```python
from build123d import *

# Parameters (mm, degrees)
ESBO_O1_W                            = 100
ESBO_O1_H                            = 40
RESSALTO_EXTRUS_O1_DEPTH             = 10
RESSALTO_EXTRUS_O2_DEPTH             = 10
ESBO_O3_W                            = 39.962527671
ESBO_O3_H                            = 3
CORTE_EXTRUS_O1_DEPTH                = 121.933866224
FILETE1_R                            = 8
FURO_DE_DI_METRO_7_0_7_1_D           = 7
FURO_DE_DI_METRO_7_0_7_1_CSINK_D     = 7.05
FURO_DE_DI_METRO_7_0_7_1_CSINK_ANGLE = 90
FURO_DE_DI_METRO_7_0_7_3_D           = 7
FURO_DE_DI_METRO_7_0_7_3_CSINK_D     = 7.05
FURO_DE_DI_METRO_7_0_7_3_CSINK_ANGLE = 90
FILETE3_R                            = 3


with BuildPart() as part:
    # Esboço1 → Ressalto-extrusão1 (new body)
    with BuildSketch(Plane(origin=(0, 0, 0), x_dir=(1, 0, 0), z_dir=(0, 1, 0))):
        with Locations((50, 20)):
            Rectangle(ESBO_O1_W, ESBO_O1_H)
    extrude(amount=RESSALTO_EXTRUS_O1_DEPTH)

    # Esboço2 → Ressalto-extrusão2 (add)
    with BuildSketch(Plane.XY):
        with BuildLine():
            Line((30, 0), (30, 35))
            ThreePointArc((30, 35), (50, 55), (70, 35))
            Line((70, 35), (70, 0))
            Line((70, 0), (30, 0))
        make_face()
    extrude(amount=-RESSALTO_EXTRUS_O2_DEPTH)

    # Esboço3 → Corte-extrusão1 (cut, through all)
    with BuildSketch(Plane.XY):
        with Locations((50.018736164, 1.5)):
            Rectangle(ESBO_O3_W, ESBO_O3_H)
    extrude(amount=-CORTE_EXTRUS_O1_DEPTH, mode=Mode.SUBTRACT)

    # Filete1
    # the kernel refuses this fillet: 8 mm, written as the material it adds along each edge
    with BuildSketch(Plane(origin=(70, 3, 0), x_dir=(-1, 0, 0), z_dir=(0, 0, -1))) as filete1_piece_1:
        with BuildLine():
            CenterArc((6.244997998, -8), FILETE1_R, 90, 51.317812547)
            Line((0, -3), (0, 0))
            Line((0, 0), (6.244997998, 0))
        make_face()
    extrude(amount=40)
    with BuildSketch(Plane(origin=(30.037472329, 3, 0), x_dir=(0, -1, 0), z_dir=(0, 0, -1))) as filete1_piece_2:
        with BuildLine():
            CenterArc((8, -6.244997998), FILETE1_R, 128.682187453, 51.317812547)
            Line((0, -6.244997998), (0, 0))
            Line((0, 0), (3, 0))
        make_face()
    extrude(amount=40)
    # the kernel refuses this fillet: 8 mm, written as the material it takes off along each edge
    with BuildSketch(Plane(origin=(100, -20, 0), x_dir=(-1, 0, 0), z_dir=(0, 1, 0)), Plane(origin=(100, -20, -40), x_dir=(0, 0, 1), z_dir=(0, 1, 0))) as filete1_2_piece_1:
        with BuildLine():
            CenterArc((FILETE1_R, -FILETE1_R), FILETE1_R, 90, 90)
            Line((0, -FILETE1_R), (0, 0))
            Line((0, 0), (FILETE1_R, 0))
        make_face()
    extrude(amount=50, mode=Mode.SUBTRACT)
    with BuildSketch(Plane(origin=(0, -20, -40), x_dir=(0, 0, 1), z_dir=(0, 1, 0)), Plane(origin=(0, -20, 0), x_dir=(1, 0, 0), z_dir=(0, 1, 0))) as filete1_2_piece_2:
        with BuildLine():
            CenterArc((FILETE1_R, FILETE1_R), FILETE1_R, 180, 90)
            Line((0, FILETE1_R), (0, 0))
            Line((0, 0), (FILETE1_R, 0))
        make_face()
    extrude(amount=50, mode=Mode.SUBTRACT)

    # Furo de diâmetro Ø7.0 (7)1 (through all)
    with Locations(Plane(origin=(0, 10, 0), x_dir=(1, 0, 0), z_dir=(0, 1, 0))):
        with Locations((8, 32)):
            CounterSinkHole(FURO_DE_DI_METRO_7_0_7_1_D / 2, FURO_DE_DI_METRO_7_0_7_1_CSINK_D / 2, counter_sink_angle=FURO_DE_DI_METRO_7_0_7_1_CSINK_ANGLE)

    # Furo de diâmetro Ø7.0 (7)3 (through all)
    with Locations(Plane(origin=(0, 10, 0), x_dir=(1, 0, 0), z_dir=(0, 1, 0))):
        with Locations((92, 32)):
            CounterSinkHole(FURO_DE_DI_METRO_7_0_7_3_D / 2, FURO_DE_DI_METRO_7_0_7_3_CSINK_D / 2, counter_sink_angle=FURO_DE_DI_METRO_7_0_7_3_CSINK_ANGLE)

    # Esboço16 → Rebaixo para parafuso de cabeça sextavada de M81 (revolve, cut)
    with BuildSketch(Plane(origin=(50, 35, 0), x_dir=(0, -1, 0), z_dir=(1, 0, 0))):
        Polygon((0, 0), (0, 40), (4.5, 40), (4.5, 5.68), (9.005, 5.68), (9.005, 0.025), (9.03, 0), align=None)
    revolve(axis=Axis((50, 35, 6.35), (0, 0, -1)), mode=Mode.SUBTRACT)

    # Filete3
    filete3_edges = [part.edges().sort_by_distance(p)[0] for p in [
        (81, 10, 0),
        (30, 22.5, -10),
        (70, 22.5, -10),
        (30, 22.5, 0),
        (70, 22.5, 0),
        (50, 55, 0),
        (50, 55, -10),
        (100, 10, -20),
        (19, 10, 0),
        (50, 10, -40),
        (0, 10, -20),
        (2.343145751, 10, -2.343145751),
        (2.343145751, 10, -37.656854249),
        (97.656854249, 10, -37.656854249),
        (97.656854249, 10, -2.343145751),
    ]]
    fillet(filete3_edges, radius=FILETE3_R)


solid = part.part
```
Design review of the part built by this model. Coordinates are the model's own, in mm. A direction names the side the tool comes from. Coordinates: 2 decimals unless noted, no trailing zeros. Order: outer loops, then holes, each group sorted by start corner. A loop starts at its lowest first (then second) coordinate and runs counter-clockwise, first axis right, second up.
1) Clearance check with flat-ended pins moving along their axes: pin 1 (10 mm diameter, centred on y = 30, z = -9.5, fed in from -X); pin 2 (11.5 mm diameter, centred on x = 50, y = 35, fed in from -Z); pin 3 (1 mm diameter, centred on x = 75.5, z = -8, fed in from +Y). State where each tip first meets the part, or that it passes through.
2) Take a section at C-C, the plane x = 15. Give the boundary of the cut face in (y, z), and give its area (3 significant figures).
3) Wall thickness on line 1 along Z through (x, y) = (8, 3.5); line 2 along X through (y, z) = (35.5, -4); line 3 along Y through (x, z) = (50, -3) (3 decimals): over which ranges is each line inside the solid? List them lowest first.
4) For faces 1 (the cylindrical face through (30.86, 22.68, -9.1)), 2 (the flat face through (54, 39, -5.68)), 3 (the flat face through (50, 3, -20)), 4 (the cylindrical face through (79.68, 9.1, -0.86)), 5 (the cylindrical face through (49.41, 9.1, -39.14)), list the 3-axis set-ups (+Z, -Z, +X, -X, +Y, -Y) from which the entire face can be reached by the end or side of a thin tool; tool diameter is ignored.
5) Take a section at D-D, the plane z = -31. State how many separate pieces and enclosed holes the cut face has, and give its area (3 significant figures).
6) Take a section at B-B, the plane z = -25.5. Give the boundary of the cut face in (x, y) (3 decimals), and give its area (3 significant figures).
7) Mouldability with a two-part tool opening along X and no side actions: class faces 6 (the cylindrical face through (57.989, 30.845, -2.813)), 7 (the cylindrical face through (67.174, 2.233, -19.72)), 8 (the cylindrical face through (30.9, 21.2, -0.86)), 9 (the flat face through (49, 10, -20)) as +X half, -X half, draft (parallel to the pull), parting line (faces both ways), or undercut.
8) Take a section at A-A, the plane x = 50. Give the boundary of the cut face in (y, z) (3 decimals), and give its area (3 significant figures).
Returned:
1. pin 1: stops at x = 30
1. pin 2: stops at z = -10
1. pin 3: stops at y = 10
2. outline: (0, -40) - (7, -40) arc R3 ccw to (10, -37) - (10, -3) arc R3 ccw to (7, 0) - (0, 0) - close
2. area: 396 mm2
3. line 1: z = -40 to -35.5, -28.5 to 0
3. line 2: x = 30.01 to 41.01, 58.99 to 69.99
3. line 3: y = 3 to 25.995, 44.005 to 55
4. face 1: -Z, -X, +Y
4. face 2: +Z
4. face 3: +Z, -Z, -Y
4. face 4: +Z, +X, +Y
4. face 5: -Z, +X, -X, +Y
5. separate pieces: 3
5. enclosed holes: 0
5. area: 753 mm2
6. outline: (0, 0) - (30.037, 0) arc R8 cw to (36.282, 3) - (63.755, 3) arc R8 cw to (70, 0) - (100, 0) - (100, 7) arc R3 ccw to (97, 10) - (3, 10) arc R3 ccw to (0, 7) - close
6. area: 888 mm2
7. face 6: undercut
7. face 7: undercut
7. face 8: -X half
7. face 9: draft
8. outline: (3, -40) - (7, -40) arc R3 ccw to (10, -37) - (10, -10) - (30.5, -10) - (30.5, -5.68) - (25.995, -5.68) - (25.995, -0.025) - (25.97, 0) - (3, 0) - close; (39.5, -10) - (52, -10) arc R3 ccw to (55, -7) - (55, -3) arc R3 ccw to (52, 0) - (44.03, 0) - (44.005, -0.025) - (44.005, -5.68) - (39.5, -5.68) - close
8. area: 583 mm2
